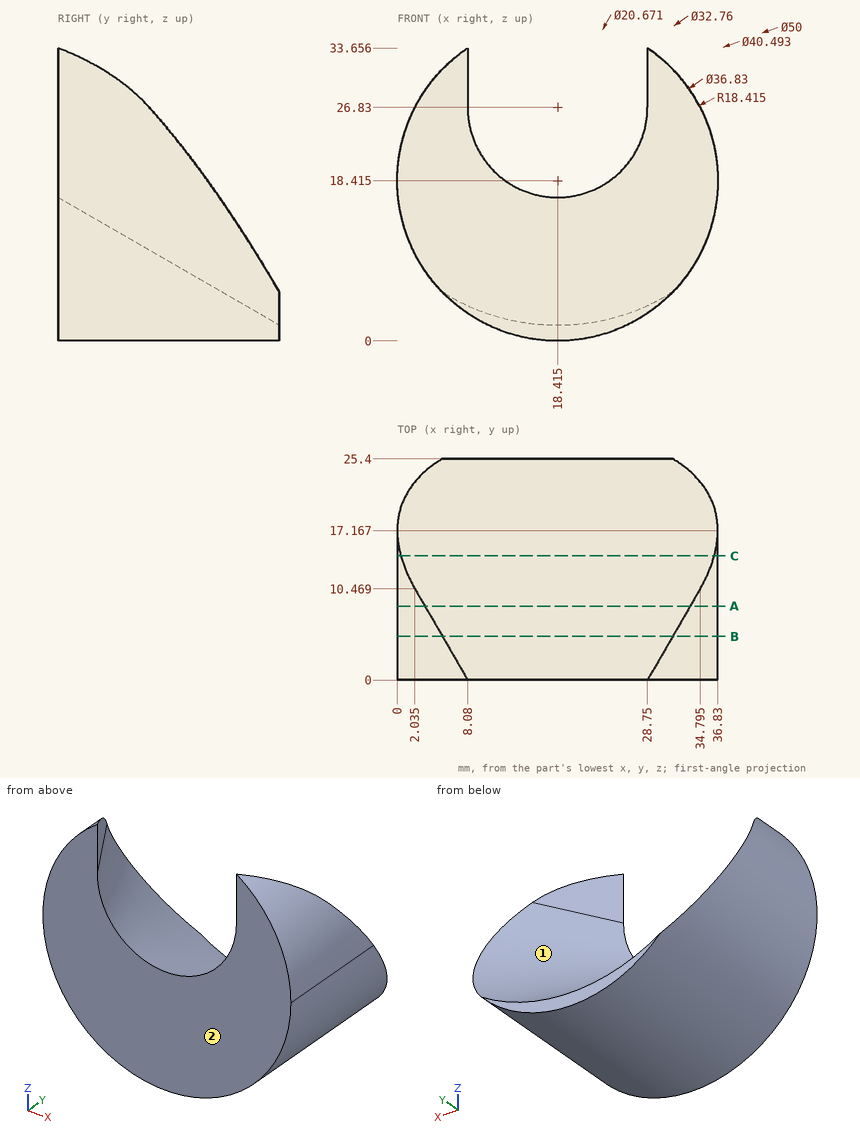
Drawing for the job (mm, zero at the part's lowest x, y, z). Coordinates: 2 decimals unless noted, no trailing zeros. Order: outer loops, then holes, each group sorted by start corner. A loop starts at its lowest first (then second) coordinate and runs counter-clockwise, first axis right, second up. Notation, with made-up numbers: (7, 34) - (51, 34) arc R15 ccw to (51, 60) - close; hole circle Ø6 at (55.25, 63.5). An arc over 180 degrees is marked (long way). Use a Markdown table: item, result. Add a question column.
(1) Saw through at B-B (y = 5). Give the cut face in (x, z) (1 decimal), then the cut area to 3 significant figures.
(2) Saw through at C-C (y = 14.25). Give the cut face in (x, z) (1 decimal), then the cut area to 3 significant figures.
(3) Pull direction X, two halves, no side cores. Call the marked faces 1 and 2: +X half, -X half, draft (parallel to the pull), parting line (faces both ways), or undercut.
(4) Flat gauge pins, fed straight in: pin 1 (1.5 mm diameter, centred on y = 17, z = 5.5, fed in from +X); pin 2 (2 mm diameter, centred on x = 27.5, z = 13, fed in from +Y); pin 3 (1.5 mm diameter, centred on x = 20, y = 8.5, fed in from +Z). Where does each tip first touch, or does it go through?
(5) Drill centre lines: line 1 along X through (y, z) = (7, 29) (1 decimal); line 2 along X through (y, z) = (3.5, 18.5); line 3 along Y through (x, z) = (32, 29.5) (1 decimal). Where is each one in solid material? Low to high. Write a range as [from, to].
(6) Saw through at A-A (y = 8.5). Give the cut face in (x, z) (1 decimal), then the cut area to 3 significant figures.
Solved:
| question | item | result |
|---|---|---|
| 1 | outline | (5.2, 26.8) - (5.2, 31.2) arc R18.4 ccw (long way) to (31.6, 31.2) - (31.6, 26.8) arc R13.2 cw to start |
| 1 | area | 572 mm² |
| 2 | outline | (0.4, 22.3) arc R18.4 ccw (long way) to (36.4, 22.3) arc R18.6 cw to start |
| 2 | area | 300 mm² |
| 3 | face 1 | undercut |
| 3 | face 2 | draft |
| 4 | pin 1 | stops at x = 32.24 |
| 4 | pin 2 | stops at y = 12.49 |
| 4 | pin 3 | stops at z = 12.11 |
| 5 | line 1 | x = [3.3, 4], [32.8, 33.5] |
| 5 | line 2 | x = [0, 9.29], [27.54, 36.83] |
| 5 | line 3 | y = [0, 5.6] |
| 6 | outline | (3.2, 26.8) - (3.2, 28.7) arc R18.4 ccw (long way) to (33.7, 28.7) - (33.7, 26.8) arc R15.2 cw to start |
| 6 | area | 469 mm² |
